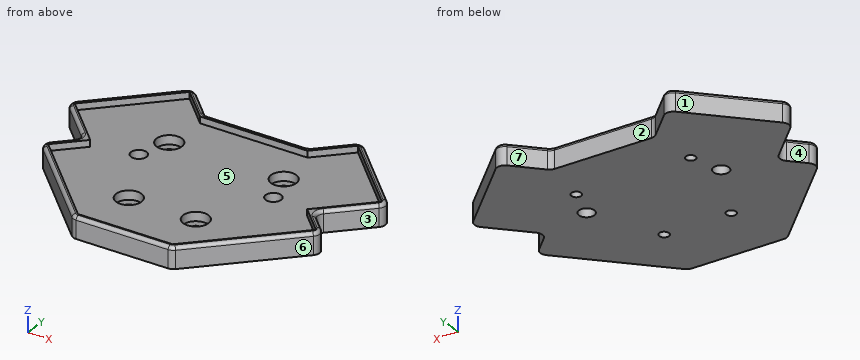
from build123d import *

# Parameters (mm, degrees)
F2_R     = 7.75
F2_R_2   = 4.75
F3_DEPTH = 9
F4_DEPTH = 13
F0_R     = 7.75
F0_R_2   = 3
F5_DEPTH = 3.5
F6_R     = 5
F7_R     = 2


with BuildPart() as f3:
    # F2 (on Top) → F3 (new body)
    with BuildSketch(Plane.XY):
        Polygon((32.864719, 52.628166), (0, 52.628166), (-32.864719, 52.628166), (-51.497475, 71.260922), (-93.923882, 28.834515), (-66.346717, 1.25735), (-81.903066, -14.298999), (-28.980231, -67.221834), (0, -67.221834), (28.980231, -67.221834), (81.903066, -14.298999), (66.346717, 1.25735), (93.923882, 28.834515), (51.497475, 71.260922), align=None)
        with Locations((-20.5, -32.721834)):
            Circle(F2_R, mode=Mode.SUBTRACT)
        with Locations((20.5, -32.721834)):
            Circle(F2_R, mode=Mode.SUBTRACT)
        with Locations((-41.15, 8.128166)):
            Circle(F2_R_2, mode=Mode.SUBTRACT)
        with Locations((-35, 27.128166)):
            Circle(F2_R, mode=Mode.SUBTRACT)
        with Locations((41.15, 8.128166)):
            Circle(F2_R_2, mode=Mode.SUBTRACT)
        with Locations((35, 27.128166)):
            Circle(F2_R, mode=Mode.SUBTRACT)
    extrude(amount=F3_DEPTH)

    # F2 (on Top) → F4 (join)
    with BuildSketch(Plane.XY):
        Polygon((0, 55.628166), (-31.622078, 55.628166), (-51.497475, 75.503562), (-98.166522, 28.834515), (-70.589358, 1.25735), (-86.145707, -14.298999), (-30.222871, -70.221834), (0, -70.221834), (30.222871, -70.221834), (86.145707, -14.298999), (70.589358, 1.25735), (98.166522, 28.834515), (51.497475, 75.503562), (31.622078, 55.628166), align=None)
        Polygon((-32.864719, 52.628166), (0, 52.628166), (32.864719, 52.628166), (51.497475, 71.260922), (93.923882, 28.834515), (66.346717, 1.25735), (81.903066, -14.298999), (28.980231, -67.221834), (0, -67.221834), (-28.980231, -67.221834), (-81.903066, -14.298999), (-66.346717, 1.25735), (-93.923882, 28.834515), (-51.497475, 71.260922), align=None, mode=Mode.SUBTRACT)
    extrude(amount=F4_DEPTH)

    # F0 (on Top) → F5 (join)
    with BuildSketch(Plane.XY):
        with Locations((-35, 27.128166)):
            Circle(F0_R)
        with Locations((-35, 27.128166)):
            Circle(F0_R_2, mode=Mode.SUBTRACT)
        with Locations((35, 27.128166)):
            Circle(F0_R)
        with Locations((35, 27.128166)):
            Circle(F0_R_2, mode=Mode.SUBTRACT)
        with Locations((20.5, -32.721834)):
            Circle(F0_R)
        with Locations((20.5, -32.721834)):
            Circle(F0_R_2, mode=Mode.SUBTRACT)
        with Locations((-20.5, -32.721834)):
            Circle(F0_R)
        with Locations((-20.5, -32.721834)):
            Circle(F0_R_2, mode=Mode.SUBTRACT)
    extrude(amount=F5_DEPTH)

    # F6
    f6_edges = [f3.edges().sort_by_distance(p)[0] for p in [
        (-51.497475, 75.503562, 6.5),
        (-31.622078, 55.628166, 6.5),
        (51.497475, 75.503562, 6.5),
        (98.166522, 28.834515, 6.5),
        (70.589358, 1.25735, 6.5),
        (86.145707, -14.298999, 6.5),
        (30.222871, -70.221834, 6.5),
        (-30.222871, -70.221834, 6.5),
        (-86.145707, -14.298999, 6.5),
        (-70.589358, 1.25735, 6.5),
        (-98.166522, 28.834515, 6.5),
        (31.622078, 55.628166, 6.5),
    ]]
    fillet(f6_edges, radius=F6_R)

    # F7
    f7_edges = [f3.edges().sort_by_distance(p)[0] for p in [
        (-74.831998, 52.169039, 13),
        (-40.524242, 64.53033, 13),
        (0, 55.628166, 13),
        (40.524242, 64.53033, 13),
        (74.831998, 52.169039, 13),
        (84.37794, 15.045933, 13),
        (78.367532, -6.520824, 13),
        (57.148755, -43.295951, 13),
        (0, -70.221834, 13),
        (-57.148755, -43.295951, 13),
        (-78.367532, -6.520824, 13),
        (-84.37794, 15.045933, 13),
    ]]
    fillet(f7_edges, radius=F7_R)


solid = f3.part
Geometry check sheet. Reference: the model listing, model coordinates, mm. Face numbers are marked on the shaded views. A direction names the side the tool comes from. Round coordinates to 2 decimals unless told otherwise and drop trailing zeros. Loops run counter-clockwise (first coordinate to the right, second up) from the corner with the lowest first, then second, coordinate; pieces in that order, holes last.
Item 1: Mould release check, pull along X, two halves, no side actions. Record for the marked faces 4, 5, 6 and 7: pulls with the +X half, pulls with the -X half, needs draft (parallel to the pull), parting line crosses it, or undercut.
Item 2: Thickness scan on line 1 (Y direction, x = -20.5, z = 2.5); line 2 (Z direction, x = -27, y = 46); line 3 (Y direction, x = 35, z = 2.7). Record the ranges inside material, lowest first.
Item 3: Cross-section at A-A on x = 20.5. Record the boundary of the cut face in (y, z).
Item 4: Access from +Z, -Z, +X, -X, +Y, -Y to the whole of each face (thin tool, end or side, straight path). Record for the marked faces 1, 2 and 3.
Item 5: Gauge pin test, flat ends, axial feed: pin 1 (11 mm diameter, centred on x = 41.15, y = 8.13, fed in from +Z); pin 2 (8 mm diameter, centred on x = -35, y = 27.13, fed in from -Z); pin 3 (3 mm diameter, centred on y = -16.5, z = 9.5, fed in from -X); pin 4 (1.2 mm diameter, centred on x = -14, z = 10.5, fed in from +Y). Record the tip position at first contact, or that the pin passes through.
Answer sheet:
1. face 4: pulls with the -X half
1. face 5: undercut
1. face 6: pulls with the +X half
1. face 7: undercut
2. line 1: y = -70.22 to -35.72, -29.72 to 55.63
2. line 2: z = 0 to 9
2. line 3: y = -65.44 to 24.13, 30.13 to 59.01
3. outline: (-70.22, 0) - (-35.72, 0) - (-35.72, 3.5) - (-40.47, 3.5) - (-40.47, 9) - (-67.22, 9) - (-67.22, 13) - (-68.22, 13) arc R2 ccw to (-70.22, 11) - close; (-29.72, 0) - (55.63, 0) - (55.63, 11) arc R2 ccw to (53.63, 13) - (52.63, 13) - (52.63, 9) - (-24.97, 9) - (-24.97, 3.5) - (-29.72, 3.5) - close
4. face 1: +Z, -Z, -X, +Y
4. face 2: +Z, -Z, +Y
4. face 3: +Z, -Z, +X
5. pin 1: stops at z = 9
5. pin 2: stops at z = 0
5. pin 3: stops at x = -84.03
5. pin 4: stops at y = 55.63
